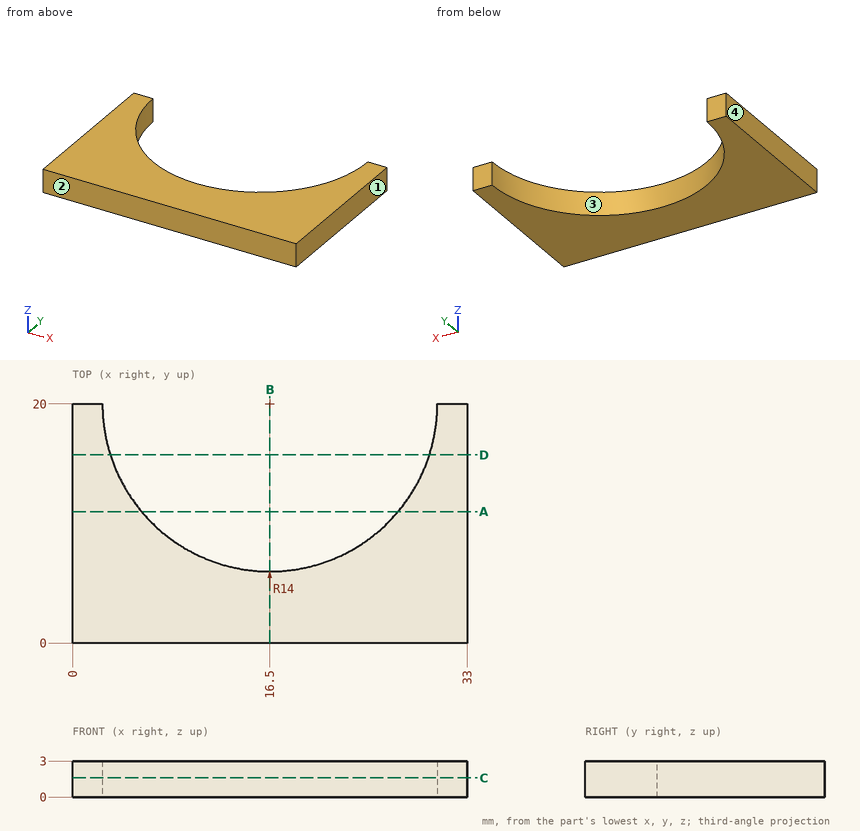
Design review of the part shown in the three views and the two pictorial views. Dimensions are in mm from the part's minimum x, y and z. Give positions to 0.01 mm unless a question says otherwise; leave off trailing zeros. Loops run counter-clockwise (first coordinate to the right, second up) from the corner with the lowest first, then second, coordinate; pieces in that order, holes last. Notation, with made-up numbers: (-27.5, -16) -> (7.5, -16) arc R21 cw to (7.5, 3) -> close; hole circle Ø7 at (34.5, 72). An arc over 180 degrees is marked (long way). Put each result on its own line as item: value. Start each with the question number.
1. We need section B-B on x = 16.5. State the section outline as (y, z) points.
2. We need section A-A on y = 11. State the section outline as (x, z) points.
3. Wall thickness on probe 1 along X at (y, z) = (9.75, 0.8); probe 2 along X at (y, z) = (19, 1); probe 3 along Y at (x, z) = (17, 1.5): over which ranges is each line inside the solid? List them lowest first.
4. Mouldability with a two-part tool opening along X and no side actions: class the marked faces 1, 2, 3 and 4 as released by +X, released by -X, zero draft, split by the parting line, or undercut.
5. We need section C-C on z = 1.6. State the section outline as (x, y) points, then the cut area to 3 significant figures.
6. We need section D-D on y = 15.75. State the section outline as (x, z) points, then the cut area to 3 significant figures.
7. Clearance check with a flat-ended pin moving along its axis: P1, Ø2, axis at x = 25.5, y = 13, coming from the +Z side. State where the tip first meets the part, or that it passes through.
Determined:
1. outline: (0, 0) -> (6, 0) -> (6, 3) -> (0, 3) -> close
2. outline: (0, 0) -> (5.78, 0) -> (5.78, 3) -> (0, 3) -> close; (27.22, 0) -> (33, 0) -> (33, 3) -> (27.22, 3) -> close
3. probe 1: 0 to 6.96, 26.04 to 33
3. probe 2: 0 to 2.54, 30.46 to 33
3. probe 3: 0 to 6.01
4. face 1: released by +X
4. face 2: zero draft
4. face 3: undercut
4. face 4: released by -X
5. outline: (0, 0) -> (33, 0) -> (33, 20) -> (30.5, 20) arc R14 cw to (2.5, 20) -> (0, 20) -> close
5. area: 352 mm^2
6. outline: (0, 0) -> (3.16, 0) -> (3.16, 3) -> (0, 3) -> close; (29.84, 0) -> (33, 0) -> (33, 3) -> (29.84, 3) -> close
6. area: 19.0 mm^2
7. P1: through
